```python
from build123d import *

# Parameters (mm, degrees)
BOSS_EXTRUDE1_DEPTH = 35
SKETCH3_W           = 44
SKETCH3_H           = 36
CUT_EXTRUDE1_DEPTH  = 90.567584934
CHAMFER1_SIZE       = 10
CHAMFER1_SIZE_2     = 11.096755526
CHAMFER1_SIZE2      = 10.174134289
CHAMFER1_SIZE2_2    = 10.73729935


with BuildPart() as part:
    # Sketch1 → Boss-Extrude1 (new, symmetric)
    with BuildSketch(Plane.XY):
        Polygon((75, 0), (-75, 0), (-75, 20), (-30.241576831, 34.239630123), (75, 15), align=None)
    extrude(amount=BOSS_EXTRUDE1_DEPTH, both=True)

    # Sketch3 → Cut-Extrude1 (cut, through all)
    with BuildSketch(Plane.XZ):
        Polygon((-30.49, 35), (75, 25), (75, 35), align=None)
        Polygon((75, -35), (75, -25), (-30.49, -35), align=None)
        with Locations((-53, 0)):
            Rectangle(SKETCH3_W, SKETCH3_H)
        Polygon((-75, 25), (-30.49, 35), (-75, 35), align=None)
        Polygon((-75, -35), (-30.49, -35), (-75, -25), align=None)
    extrude(amount=-CUT_EXTRUDE1_DEPTH, mode=Mode.SUBTRACT)

    # Chamfer1
    chamfer1_edges = [part.edges().sort_by_distance(p)[0] for p in [
        (-52.745, 0, 30),
    ]]
    chamfer(chamfer1_edges, length=CHAMFER1_SIZE)
    chamfer1_2_edges = [part.edges().sort_by_distance(p)[0] for p in [
        (-52.745, 0, -30),
    ]]
    chamfer(chamfer1_2_edges, length=CHAMFER1_SIZE)
    chamfer1_3_edges = [part.edges().sort_by_distance(p)[0] for p in [
        (75, 7.5, 25),
    ]]
    chamfer1_3_side = [part.faces().sort_by_distance(p)[0] for p in [
        (75, 7.5, 24.8),
    ]]
    chamfer(chamfer1_3_edges, length=CHAMFER1_SIZE_2, length2=CHAMFER1_SIZE, reference=chamfer1_3_side[0])
    chamfer1_4_edges = [part.edges().sort_by_distance(p)[0] for p in [
        (75, 7.5, -25),
    ]]
    chamfer1_4_side = [part.faces().sort_by_distance(p)[0] for p in [
        (75, 7.5, -24.8),
    ]]
    chamfer(chamfer1_4_edges, length=CHAMFER1_SIZE, length2=CHAMFER1_SIZE_2, reference=chamfer1_4_side[0])
    chamfer1_5_edges = [part.edges().sort_by_distance(p)[0] for p in [
        (17.401526868, 25.52980535, 30.460088457),
    ]]
    chamfer1_5_side = [part.faces().sort_by_distance(p)[0] for p in [
        (17.365875348, 25.3330376, 30.463468068),
    ]]
    chamfer(chamfer1_5_edges, length=CHAMFER1_SIZE, length2=CHAMFER1_SIZE2, reference=chamfer1_5_side[0])
    chamfer1_6_edges = [part.edges().sort_by_distance(p)[0] for p in [
        (-58.87630634, 25.129658681, 28.622487904),
    ]]
    chamfer1_6_side = [part.faces().sort_by_distance(p)[0] for p in [
        (-58.818457754, 24.938649191, 28.635484665),
    ]]
    chamfer(chamfer1_6_edges, length=CHAMFER1_SIZE, length2=CHAMFER1_SIZE2_2, reference=chamfer1_6_side[0])
    chamfer1_7_edges = [part.edges().sort_by_distance(p)[0] for p in [
        (-52.745, 27.080297874, -30),
    ]]
    chamfer1_7_side = [part.faces().sort_by_distance(p)[0] for p in [
        (-52.705100441, 27.092991685, -29.804431873),
    ]]
    chamfer(chamfer1_7_edges, length=CHAMFER1_SIZE, length2=CHAMFER1_SIZE2_2, reference=chamfer1_7_side[0])
    chamfer1_8_edges = [part.edges().sort_by_distance(p)[0] for p in [
        (23.400963602, 24.433024522, -29.891367561),
    ]]
    chamfer1_8_side = [part.faces().sort_by_distance(p)[0] for p in [
        (23.382696848, 24.43636394, -29.692231492),
    ]]
    chamfer(chamfer1_8_edges, length=CHAMFER1_SIZE, length2=CHAMFER1_SIZE2, reference=chamfer1_8_side[0])


solid = part.part
```
Part model, mm, in its own coordinate system. A direction names the side the tool comes from. Give positions to 0.01 mm unless a question says otherwise; leave off trailing zeros. Write each loop counter-clockwise with the first axis right and the second up, starting at its lowest first coordinate (ties: lowest second). Pieces come first, ordered by that corner, then holes. Notation, with made-up numbers: (-23, 68) -> (-11, 68) arc R20 cw to (-11, 106) -> close; hole circle Ø5 at (36, 3.25). An arc over 180 degrees is marked (long way). Put each result on its own line as item: value. Start each with the question number.
Item 1: Pull direction Z, two halves, no side cores. Call faces 1 (the face through (-31, 17, 0)), 2 (the face through (6.899, 9.06, -31.456)), 3 (the face through (-46.432, 5.07, 26.365)): pulls with the +Z half, pulls with the -Z half, needs draft (parallel to the pull), parting line crosses it, or undercut.
Item 2: Cut at D-D (x = -17.5). List the corners of the cut face in (y, z), then the cut area to 3 significant figures.
Item 3: Cut at A-A (x = -37.5). List the corners of the cut face in (y, z).
Item 4: Which spindle directions (+Z, -Z, +X, -X, +Y, -Y) get a long thin tool onto all of the face, cutting with end or side? Do faces 4 (the face through (-48, 13, 18)), 5 (the face through (22.727, 19.313, -25.004)). Say none if no direction does.
Item 5: Pin check, flat tips, straight feed: pin 1 Ø8 at (x, y) = (-5.5, 12) entering from +Z; pin 2 Ø2 at (x, y) = (-33.5, 4) entering from -Z; pin 3 Ø5 at (x, y) = (11, 5) entering from +Z. Stop position of each tip, or through.
Item 6: Cut at C-C (y = 28). List the corners of the cut face in (x, z).
Item 7: Cut at B-B (z = -1). List the corners of the cut face in (x, y), then the cut area to 3 significant figures.
Item 8: Wall check: L1, parallel to Z at x = -62.5, y = 20.5; L2, parallel to Z at x = -32, y = 28.5; L3, parallel to X at y = 8, z = 0. Give the ranges that are in metal, low to high. Write a range as [from, to].
Answer list:
1. face 1: undercut
1. face 2: pulls with the -Z half
1. face 3: pulls with the +Z half
2. outline: (0, -27.67) -> (5.95, -33.77) -> (21.57, -33.77) -> (31.91, -23.73) -> (31.91, 23.55) -> (21.75, 33.77) -> (5.95, 33.77) -> (0, 27.67) -> close
2. area: 2,010 mm2
3. outline: (0, -23.18) -> (10, -33.43) -> (20.69, -33.43) -> (31.93, -23.2) -> (31.93, -18) -> (0, -18) -> close; (0, 18) -> (31.93, 18) -> (31.93, 22.44) -> (21.46, 33.43) -> (10, 33.43) -> (0, 23.18) -> close
4. face 4: -X, +Y, -Y
4. face 5: -Z, +X, +Y
5. pin 1: stops at z = 33.01
5. pin 2: stops at z = -29.22
5. pin 3: stops at z = 31.3
6. outline: (-49.85, -20.42) -> (-29.62, -30.82) -> (3.89, -21.7) -> (3.89, 21.52) -> (-29.75, 30.89) -> (-49.85, 19.67) -> (-49.85, 18) -> (-31, 18) -> (-31, -18) -> (-49.85, -18) -> close
7. outline: (-31, 0) -> (75, 0) -> (75, 15) -> (-30.24, 34.24) -> (-31, 34) -> close
7. area: 2,620 mm2
8. L1: z = [-20.74, -18], [18, 20.47]
8. L2: z = [-29.15, -18], [18, 29.11]
8. L3: x = [-31, 75]
